Check sheet for the modelled part. Datum: model origin and axes. Units: mm. A direction names the side the tool comes from. Coordinates: 2 decimals unless noted, no trailing zeros. Loops run counter-clockwise (first coordinate to the right, second up) from the corner with the lowest first, then second, coordinate; pieces in that order, holes last. Notation, with made-up numbers: (-34.75, -34.75) - (-4.75, -34.75) arc R23 ccw to (-4.75, -8.75) - close; hole circle Ø4 at (18.25, -10.75). An arc over 180 degrees is marked (long way). Use a Markdown table: item, result. Add a question column.
1) Thickness scan on line 1 (Z direction, x = 26, y = 1) (3 decimals); line 2 (X direction, y = 5.6, z = 0) (3 decimals); line 3 (X direction, y = 4.15, z = 7.62) (3 decimals). Record the ranges inside material, lowest first.
2) Tool access check on faces 5 (the flat face through (-13, 3.175, 8)), 6 (the flat face through (-1, 3, 41.275)). Record the directions out of +Z, -Z, +X, -X, +Y, -Y that give a thin tool (end or side, any length) a straight path to the whole face; none if there is none.
3) Sectioned sample at A-A, the plane x = -27.94. Enter the section's corners in (y, z) (3 decimals).
4) Sectioned sample at D-D, the plane x = 0. Enter the section's corners in (y, z) (3 decimals), then the cut area to 3 significant figures.
5) Sectioned sample at B-B, the plane z = -3. Enter the section's corners in (x, y) (3 decimals).
6) Go/stop test with a flat-tipped pin: P1, Ø0.6, axis at x = -0.5, z = 15, coming from the +Y side (3 decimals). Record where the tip stops, or that it passes through.
7) Sectioned sample at C-C, the plane x = 36.5. Enter the section's corners in (y, z) (3 decimals).
8) Draft check along X on faces 1 (the cylindrical face through (-6.37, 5.87, -1.42)), 2 (the flat face through (0, 3.175, -15)), 3 (the flat face through (-41.275, 3, 1)), 4 (the flat face through (-10, 0, -1)). Enter one of: pulls with the +X half, pulls with the -X half, needs draft (parallel to the pull), parting line crosses it, or undercut.
from build123d import *

# Parameters (mm, degrees)
SKETCH1_W           = 82.55
SKETCH1_H           = 82.55
BOSS_EXTRUDE1_DEPTH = 6.35
CUT_EXTRUDE1_REACH  = 60.716
SKETCH2_R           = 4.699
SKETCH4_R           = 7.9248
SKETCH4_R_2         = 6.5278
CUT_EXTRUDE3_DEPTH  = 0.9779
SKETCH5_R           = 1.03251
CUT_EXTRUDE4_DEPTH  = 3.175
CIRPATTERN1_COUNT   = 6
CUT_EXTRUDE5_REACH  = 60.716
SKETCH6_R           = 1.63195
CIRPATTERN2_COUNT   = 9
CUT_EXTRUDE6_REACH  = 60.716
SKETCH7_R           = 3.175


with BuildPart() as part:
    # Sketch1 → Boss-Extrude1 (new body)
    with BuildSketch(Plane(origin=(0, 0, 0), x_dir=(1, 0, 0), z_dir=(0, 1, 0))):
        Rectangle(SKETCH1_W, SKETCH1_H)
    extrude(amount=BOSS_EXTRUDE1_DEPTH)

    # Sketch2 → Cut-Extrude1 (cut, up to next)
    with BuildSketch(Plane(origin=(0, 6.35, 0), x_dir=(1, 0, 0), z_dir=(0, 1, 0)), mode=Mode.PRIVATE) as cut_extrude1_sk1:
        with Locations(Location((0, 0, 0), (0, 0, 270))):
            Circle(SKETCH2_R)
    cut_extrude1_tool1 = extrude(cut_extrude1_sk1.sketch, amount=-CUT_EXTRUDE1_REACH, mode=Mode.PRIVATE) & part.part
    add(cut_extrude1_tool1.solids().sort_by_distance((0, 6.35, 0))[0], mode=Mode.SUBTRACT)

    # Sketch4 → Cut-Extrude3 (cut)
    with BuildSketch(Plane(origin=(0, 6.35, 0), x_dir=(1, 0, 0), z_dir=(0, 1, 0))):
        with Locations(Location((0, 0, 0), (0, 0, 270))):
            Circle(SKETCH4_R)
        with Locations(Location((0, 0, 0), (0, 0, 270))):
            Circle(SKETCH4_R_2, mode=Mode.SUBTRACT)
    extrude(amount=-CUT_EXTRUDE3_DEPTH, mode=Mode.SUBTRACT)

    # Sketch5 → Cut-Extrude4 (cut)
    with BuildSketch(Plane(origin=(0, 6.35, 0), x_dir=(1, 0, 0), z_dir=(0, 1, 0))):
        with Locations(Location((0, -15.24, 0), (0, 0, 270))):
            Circle(SKETCH5_R)
    cut_extrude4 = extrude(amount=-CUT_EXTRUDE4_DEPTH, mode=Mode.SUBTRACT)

    # CirPattern1: Cut-Extrude4 ×6 about axis
    cirpattern1_axis = Axis((0, 0, 0), (0, 1, 0))
    for i in range(1, CIRPATTERN1_COUNT):
        add(cut_extrude4.rotate(cirpattern1_axis, i * 360 / CIRPATTERN1_COUNT), mode=Mode.SUBTRACT)

    # Sketch6 → Cut-Extrude5 (cut, up to next)
    with BuildSketch(Plane(origin=(0, 6.35, 0), x_dir=(1, 0, 0), z_dir=(0, 1, 0)), mode=Mode.PRIVATE) as cut_extrude5_sk1:
        with Locations(Location((13.97, -24.196749782, 0), (0, 0, 270))):
            Circle(SKETCH6_R)
    cut_extrude5_tool1 = extrude(cut_extrude5_sk1.sketch, amount=-CUT_EXTRUDE5_REACH, mode=Mode.PRIVATE) & part.part
    cut_extrude5 = cut_extrude5_tool1.solids().sort_by_distance((13.97, 6.35, 24.19675))[0]
    add(cut_extrude5, mode=Mode.SUBTRACT)

    # CirPattern2: Cut-Extrude5 ×9 about axis
    cirpattern2_axis = Axis((0, 0, 0), (0, 1, 0))
    for i in range(1, CIRPATTERN2_COUNT):
        add(cut_extrude5.rotate(cirpattern2_axis, i * 360 / CIRPATTERN2_COUNT), mode=Mode.SUBTRACT)

    # Sketch7 → Cut-Extrude6 (cut, up to next)
    with BuildSketch(Plane(origin=(0, 6.35, 0), x_dir=(1, 0, 0), z_dir=(0, 1, 0)), mode=Mode.PRIVATE) as cut_extrude6_sk1:
        with Locations(Location((34.925, 34.925, 0), (0, 0, 270))):
            Circle(SKETCH7_R)
    cut_extrude6_tool1 = extrude(cut_extrude6_sk1.sketch, amount=-CUT_EXTRUDE6_REACH, mode=Mode.PRIVATE) & part.part
    # Sketch7 → Cut-Extrude6 (cut, up to next)
    with BuildSketch(Plane(origin=(0, 6.35, 0), x_dir=(1, 0, 0), z_dir=(0, 1, 0)), mode=Mode.PRIVATE) as cut_extrude6_sk2:
        with Locations(Location((34.925, -34.925, 0), (0, 0, 90))):
            Circle(SKETCH7_R)
    cut_extrude6_tool2 = extrude(cut_extrude6_sk2.sketch, amount=-CUT_EXTRUDE6_REACH, mode=Mode.PRIVATE) & part.part
    # Sketch7 → Cut-Extrude6 (cut, up to next)
    with BuildSketch(Plane(origin=(0, 6.35, 0), x_dir=(1, 0, 0), z_dir=(0, 1, 0)), mode=Mode.PRIVATE) as cut_extrude6_sk3:
        with Locations(Location((-34.925, -34.925, 0), (0, 0, 270))):
            Circle(SKETCH7_R)
    cut_extrude6_tool3 = extrude(cut_extrude6_sk3.sketch, amount=-CUT_EXTRUDE6_REACH, mode=Mode.PRIVATE) & part.part
    # Sketch7 → Cut-Extrude6 (cut, up to next)
    with BuildSketch(Plane(origin=(0, 6.35, 0), x_dir=(1, 0, 0), z_dir=(0, 1, 0)), mode=Mode.PRIVATE) as cut_extrude6_sk4:
        with Locations(Location((-34.925, 34.925, 0), (0, 0, 90))):
            Circle(SKETCH7_R)
    cut_extrude6_tool4 = extrude(cut_extrude6_sk4.sketch, amount=-CUT_EXTRUDE6_REACH, mode=Mode.PRIVATE) & part.part
    add(cut_extrude6_tool1.solids().sort_by_distance((34.925, 6.35, -34.925))[0], mode=Mode.SUBTRACT)
    add(cut_extrude6_tool2.solids().sort_by_distance((34.925, 6.35, 34.925))[0], mode=Mode.SUBTRACT)
    add(cut_extrude6_tool3.solids().sort_by_distance((-34.925, 6.35, 34.925))[0], mode=Mode.SUBTRACT)
    add(cut_extrude6_tool4.solids().sort_by_distance((-34.925, 6.35, -34.925))[0], mode=Mode.SUBTRACT)


solid = part.part
Solved:
| question | item | result |
|---|---|---|
| 1 | line 1 | z = -41.275 to -11.168, -7.944 to 7.944, 11.168 to 41.275 |
| 1 | line 2 | x = -41.275 to -29.572, -26.308 to -7.925, -6.528 to -4.699, 4.699 to 6.528, 7.925 to 41.275 |
| 1 | line 3 | x = -41.275 to -14.231, -12.166 to 12.166, 14.231 to 41.275 |
| 2 | face 5 | +Y |
| 2 | face 6 | +Z, +X, -X, +Y, -Y |
| 3 | outline | (0, -41.275) - (6.35, -41.275) - (6.35, -1.632) - (0, -1.632) - close; (0, 1.632) - (6.35, 1.632) - (6.35, 41.275) - (0, 41.275) - close |
| 4 | outline | (0, -41.275) - (6.35, -41.275) - (6.35, -16.273) - (3.175, -16.273) - (3.175, -14.207) - (6.35, -14.207) - (6.35, -7.925) - (5.372, -7.925) - (5.372, -6.528) - (6.35, -6.528) - (6.35, -4.699) - (0, -4.699) - close; (0, 4.699) - (6.35, 4.699) - (6.35, 6.528) - (5.372, 6.528) - (5.372, 7.925) - (6.35, 7.925) - (6.35, 14.207) - (3.175, 14.207) - (3.175, 16.273) - (6.35, 16.273) - (6.35, 41.275) - (0, 41.275) - close |
| 4 | area | 449 mm2 |
| 5 | outline | (-41.275, 0) - (-3.617, 0) - (-3.617, 6.35) - (-5.798, 6.35) - (-5.798, 5.372) - (-7.335, 5.372) - (-7.335, 6.35) - (-41.275, 6.35) - close; (3.617, 0) - (41.275, 0) - (41.275, 6.35) - (7.335, 6.35) - (7.335, 5.372) - (5.798, 5.372) - (5.798, 6.35) - (3.617, 6.35) - close |
| 6 | P1 | stops at y = 3.175 |
| 7 | outline | (0, -41.275) - (6.35, -41.275) - (6.35, -37.682) - (0, -37.682) - close; (0, -32.168) - (6.35, -32.168) - (6.35, 32.168) - (0, 32.168) - close; (0, 37.682) - (6.35, 37.682) - (6.35, 41.275) - (0, 41.275) - close |
| 8 | face 1 | undercut |
| 8 | face 2 | undercut |
| 8 | face 3 | pulls with the -X half |
| 8 | face 4 | needs draft |
